from build123d import *

# Parameters (mm, degrees)
EXTRUDE_1_DEPTH     = 48
FILLET_1_R          = 24
FILLET_2_R          = 24
FILLET_3_R          = 24
FILLET_4_R          = 24
SKETCH_8_W          = 46
SKETCH_8_H          = 25
CUT_EXTRUDE_2_DEPTH = 134.701159307
SKETCH_9_R          = 5.1
CUT_EXTRUDE_3_DEPTH = 48
SKETCH_11_R         = 8.25
CUT_EXTRUDE_4_DEPTH = 18
SKETCH_12_R         = 15
CUT_EXTRUDE_5_DEPTH = 7


with BuildPart() as part:
    # Эскиз1 → Бобышка-Вытянуть1 (new body)
    with BuildSketch(Plane.XY):
        Polygon((0, 0), (24, 0), (24, -4), (92, -4), (92, 0), (116, 0), (116, 8), (89, 8), (89, 46), (27, 46), (27, 8), (0, 8), align=None)
    extrude(amount=EXTRUDE_1_DEPTH)

    # Скругление1
    fillet_1_edges = [part.edges().sort_by_distance(p)[0] for p in [
        (0, 4, 48),
    ]]
    fillet(fillet_1_edges, radius=FILLET_1_R)

    # Скругление2
    fillet_2_edges = [part.edges().sort_by_distance(p)[0] for p in [
        (0, 4, 0),
    ]]
    fillet(fillet_2_edges, radius=FILLET_2_R - 0.0001)  # a hair under: the kernel refuses the full size

    # Скругление3
    fillet_3_edges = [part.edges().sort_by_distance(p)[0] for p in [
        (116, 4, 0),
    ]]
    fillet(fillet_3_edges, radius=FILLET_3_R)

    # Скругление4
    fillet_4_edges = [part.edges().sort_by_distance(p)[0] for p in [
        (116, 4, 48),
    ]]
    fillet(fillet_4_edges, radius=FILLET_4_R - 0.0001)  # a hair under: the kernel refuses the full size

    # Эскиз8 → Вырез-Вытянуть2 (cut, through all)
    with BuildSketch(Plane.XY.offset(48)):
        with Locations((58, 26.5)):
            Rectangle(SKETCH_8_W, SKETCH_8_H)
    extrude(amount=-CUT_EXTRUDE_2_DEPTH, mode=Mode.SUBTRACT)

    # Эскиз9 → Вырез-Вытянуть3 (cut)
    with BuildSketch(Plane.XZ.offset(4)):
        with Locations(Location((12.743315918, 24, 0), (0, 0, 270))):
            Circle(SKETCH_9_R)
        with Locations((102.743315918, 24)):
            Circle(SKETCH_9_R)
    extrude(amount=-CUT_EXTRUDE_3_DEPTH, mode=Mode.SUBTRACT)

    # Эскиз11 → Вырез-Вытянуть4 (cut)
    with BuildSketch(Plane.XZ.offset(4)):
        with Locations(Location((58, 24, 0), (0, 0, 270))):
            Circle(SKETCH_11_R)
    extrude(amount=-CUT_EXTRUDE_4_DEPTH, mode=Mode.SUBTRACT)

    # Эскиз12 → Вырез-Вытянуть5 (cut)
    with BuildSketch(Plane(origin=(0, 46, 0), x_dir=(1, 0, 0), z_dir=(0, 1, 0))):
        with Locations(Location((58, -24, 0), (0, 0, 180))):
            Circle(SKETCH_12_R)
    extrude(amount=-CUT_EXTRUDE_5_DEPTH, mode=Mode.SUBTRACT)


solid = part.part
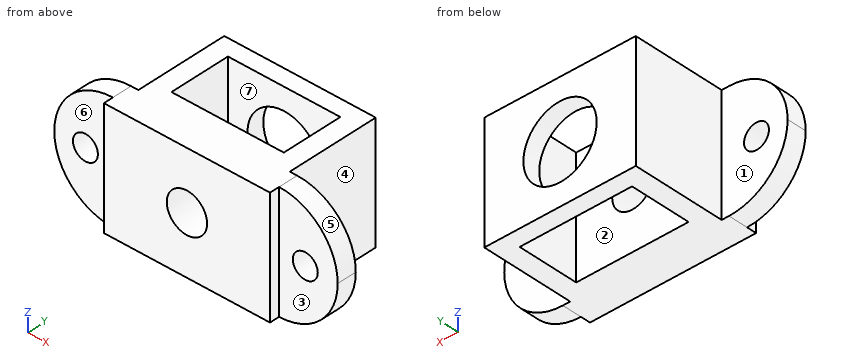
The listing builds one solid part. Answer for the finished solid, in the listing's coordinates (mm). Face numbers are marked on the shaded views. A direction names the side the tool comes from. Round coordinates to 2 decimals unless told otherwise and drop trailing zeros. Write each loop counter-clockwise with the first axis right and the second up, starting at its lowest first coordinate (ties: lowest second). Pieces come first, ordered by that corner, then holes. Notation, with made-up numbers: (-2.5, 38) - (11.5, 38) arc R24 ccw to (11.5, 66) - close; hole circle Ø4 at (28, 86). An arc over 180 degrees is marked (long way). Use a Markdown table: item, result. Add a question column.
1. The part is cut by section B-B (y = 35). Write down the section's boundary in (x, z), and give its area (3 significant figures).
2. Flat-ended cylindrical pins translate along their axes: P1, Ø4.5, axis at y = -1.5, z = 14, coming from the +X side; P2, Ø3, axis at y = 2, z = 34, coming from the -X side; P3, Ø4.5, axis at y = -3, z = 34, coming from the -X side. Find the tip coordinate at first contact, or state that the pin passes through.
3. The part is cut by section C-C (z = 17). Write down the section's boundary in (x, y).
4. The part is cut by section A-A (x = 58). Write down the section's boundary in (y, z), and give its area (3 significant figures).
5. For a pull along Y with two mould halves and no side action, classify the marked faces 5, 6 and 7 as +Y half, -Y half, draft (parallel to the pull), parting line (faces both ways), or undercut.
6. Consider line 1 (Y direction, x = 67, z = 11.5); line 2 (X direction, y = -0.25, z = 24); line 3 (X direction, y = 1, z = 21.5). Determine where each line is inside the solid, lowest interval first.
7. A tool of negligible diameter and unlimited length cuts with its end or side. For the marked faces 1, 2, 3 and 4, from which of +Z, -Z, +X, -X, +Y, -Y can it reach the whole face along a straight path? Write none if from no direction.
8. The part is cut by section D-D (y = 41). Write down the section's boundary in (x, z).
Reported:
| question | item | result |
|---|---|---|
| 1 | outline | (27, 0) - (35, 0) - (35, 48) - (27, 48) - close; (81, 0) - (89, 0) - (89, 48) - (81, 48) - close |
| 1 | area | 768 mm^2 |
| 2 | P1 | x = 114.51 |
| 2 | P2 | x = 1.56 |
| 2 | P3 | x = 24 |
| 3 | outline | (1.04, 0) - (24, 0) - (24, -4) - (53.63, -4) - (53.63, 14) - (35, 14) - (35, 39) - (44.73, 39) - (44.73, 46) - (27, 46) - (27, 8) - (1.04, 8) - close; (62.37, -4) - (92, -4) - (92, 0) - (114.96, 0) - (114.96, 8) - (89, 8) - (89, 46) - (71.27, 46) - (71.27, 39) - (81, 39) - (81, 14) - (62.37, 14) - close |
| 4 | outline | (-4, 0) - (14, 0) - (14, 15.75) - (-4, 15.75) - close; (-4, 32.25) - (14, 32.25) - (14, 48) - (-4, 48) - close; (39, 0) - (46, 0) - (46, 9) - (39, 9) - close; (39, 39) - (46, 39) - (46, 48) - (39, 48) - close |
| 4 | area | 693 mm^2 |
| 5 | face 5 | draft |
| 5 | face 6 | -Y half |
| 5 | face 7 | undercut |
| 6 | line 1 | -4 to 14, 39 to 46 |
| 6 | line 2 | 24 to 49.75, 66.25 to 92 |
| 6 | line 3 | 0.13 to 8.3, 17.19 to 50.14, 65.86 to 98.3, 107.19 to 115.87 |
| 7 | face 1 | +Z, -Z, -X, +Y |
| 7 | face 2 | +Z, -Z |
| 7 | face 3 | +Z, -Z, +X, -Y |
| 7 | face 4 | +Z, -Z, +X, +Y |
| 8 | outline | (27, 0) - (89, 0) - (89, 48) - (27, 48) - close; hole circle Ø30 at (58, 24) |
